Design review of the part built by this model. Coordinates are the model's own, in mm. A direction names the side the tool comes from. Give positions to 0.01 mm unless a question says otherwise; leave off trailing zeros. Write each loop counter-clockwise with the first axis right and the second up, starting at its lowest first coordinate (ties: lowest second). Pieces come first, ordered by that corner, then holes. Notation, with made-up numbers: M 31,-22.5 L 77,-22.5 A21 ccw 77,7.5 Z; hole C -32,-35 d4. An arc over 180 degrees is marked long. Answer in a Markdown table with one row per item.
```python
from build123d import *

# Parameters (mm, degrees)
F1_DEPTH = 2.5
F3_DEPTH = 65
F4_W     = 90
F4_H     = 200
F4_R     = 8.5
F5_DEPTH = 8
F6_W     = 90
F6_H     = 200
F6_R     = 8.5
F7_DEPTH = 8


with BuildPart() as f1:
    # F0 (on Front) → F1 (new body, symmetric)
    with BuildSketch(Plane.XZ):
        Polygon((1620, -310.9023153198), (0, 489.7515538394), (-1100, 0), (-1100, -85), (-1010, -85), (0, 349.7515538394), (1530, -408.8023153198), (1620, -408.8023153198), align=None)
    extrude(amount=F1_DEPTH, both=True)

    # F2 (on Front) → F3 (join, symmetric)
    with BuildSketch(Plane.XZ):
        Polygon((-1100, 8.757090228), (-1100, 0), (0, 489.7515538394), (1620, -310.9023153198), (1620, -302.1452250917), (0, 498.5086440674), align=None)
        Polygon((1530, -408.8023153198), (0, 349.7515538394), (-1010, -85), (-1100, -85), (-1100, -93), (-1010, -93), (0, 341.7515538394), (1530, -416.8023153198), (1620, -416.8023153198), (1620, -408.8023153198), align=None)
    extrude(amount=F3_DEPTH, both=True)

    # F4 (on face) → F5 (join)
    with BuildSketch(Plane(origin=(0, 0, -93), x_dir=(1, 0, 0), z_dir=(0, 0, -1))):
        with Locations((-1055, 0)):
            Rectangle(F4_W, F4_H)
        with Locations((-1035, -75)):
            Circle(F4_R, mode=Mode.SUBTRACT)
        with Locations((-1035, 75)):
            Circle(F4_R, mode=Mode.SUBTRACT)
    extrude(amount=-F5_DEPTH)

    # F6 (on face) → F7 (join)
    with BuildSketch(Plane(origin=(0, 0, -416.8023153198), x_dir=(1, 0, 0), z_dir=(0, 0, -1))):
        with Locations((1575, 0)):
            Rectangle(F6_W, F6_H)
        with Locations((1555, -75)):
            Circle(F6_R, mode=Mode.SUBTRACT)
        with Locations((1555, 75)):
            Circle(F6_R, mode=Mode.SUBTRACT)
    extrude(amount=-F7_DEPTH)


solid = f1.part
```
1) Add section B-B (x = 1067). Write out the cut boundary in (y, z).
Geometry says:
| item | result |
|---|---|
| outline | M -65,-187.25 L 65,-187.25 L 65,-179.25 L 2.5,-179.25 L 2.5,-37.59 L 65,-37.59 L 65,-28.84 L -65,-28.84 L -65,-37.59 L -2.5,-37.59 L -2.5,-179.25 L -65,-179.25 Z |
2) Add section C-C (z = -125). Write out the cut boundary in (x, y), and give its area (3 significant figures).
Geometry says:
| item | result |
|---|---|
| outline | M 941.44,-65 L 957.57,-65 L 957.57,-2.5 L 1243.86,-2.5 L 1243.86,-65 L 1261.57,-65 L 1261.57,65 L 1243.86,65 L 1243.86,2.5 L 957.57,2.5 L 957.57,65 L 941.44,65 Z |
| area | 5,830 mm^2 |
3) Add section A-A (z = 269). Write out the cut boundary in (x, y).
Geometry says:
| item | result |
|---|---|
| outline | M -515.48,-65 L -495.82,-65 L -495.82,-2.5 L -187.6,-2.5 L -187.6,-65 L -169.01,-65 L -169.01,65 L -187.6,65 L -187.6,2.5 L -495.82,2.5 L -495.82,65 L -515.48,65 Z; M 146.74,-65 L 162.88,-65 L 162.88,-2.5 L 446.66,-2.5 L 446.66,-65 L 464.38,-65 L 464.38,65 L 446.66,65 L 446.66,2.5 L 162.88,2.5 L 162.88,65 L 146.74,65 Z |
4) For faces 1 (the face through (-1056, 51, -85)), 2 (the face through (354, -2.5, 176)), 3 (the face through (-1056, -1, -93)), 4 (the face through (-497.93, 33.31, 135.42)), list the 3-axis set-ups (+Z, -Z, +X, -X, +Y, -Y) from which the entire face can be reached by the end or side of a thin tool; tool diameter is ignored.
Geometry says:
| item | result |
|---|---|
| face 1 | -X, +Y |
| face 2 | -Y |
| face 3 | -Z, -X, +Y, -Y |
| face 4 | +Y |
5) The part is to be moulded in two halves that separate along X. For faces 5 (the face through (1576, -52, -408.802)), 6 (the face through (-512.07, -0.91, 121.333)), 7 (the face through (821.34, 0.91, 92.577)), say which applies: released by +X, released by -X, zero draft, split by the parting line, or undercut.
Geometry says:
| item | result |
|---|---|
| face 5 | zero draft |
| face 6 | undercut |
| face 7 | released by +X |
6) Insertion check: P1, Ø19.5, axis at x = -1035, y = -75, coming from the -Z side; P2, Ø4, axis at y = 53, z = -130.5, coming from the -X side; P3, Ø9, axis at y = -83, z = -413, coming from the -X side. Each pin has a flat end and moves straight along its axis. Give the tip position at first contact, or say it passes through.
Geometry says:
| item | result |
|---|---|
| P1 | z = -93 |
| P2 | x = 948.5 |
| P3 | x = 1530 |
7) Add section D-D (z = 55.5). Write out the cut boundary in (x, y), and give its area (3 significant figures).
Geometry says:
| item | result |
|---|---|
| outline | M -995.01,-65 L -975.34,-65 L -975.34,-2.5 L -683.6,-2.5 L -683.6,-65 L -665.01,-65 L -665.01,65 L -683.6,65 L -683.6,2.5 L -975.34,2.5 L -975.34,65 L -995.01,65 Z; M 577.37,-65 L 593.5,-65 L 593.5,-2.5 L 878.64,-2.5 L 878.64,-65 L 896.36,-65 L 896.36,65 L 878.64,65 L 878.64,2.5 L 593.5,2.5 L 593.5,65 L 577.37,65 Z |
| area | 12,300 mm^2 |
8) To check wall thickness, follow probe 1 along Y at (x, z) = (-1035, -90.25); probe 2 along X at (y, z) = (75, -414.75); probe 3 along X at (y, z) = (-4.5, 133). State the ranges of each line that lie inside material, in increasing order. Write a range as [from, to].
Geometry says:
| item | result |
|---|---|
| probe 1 | [-100, -83.5], [-66.5, 66.5], [83.5, 100] |
| probe 2 | [1530, 1546.5], [1563.5, 1620] |
| probe 3 | [-820.95, -801.28], [-503.55, -484.96], [421.05, 437.19], [721.83, 739.55] |
